```python
from build123d import *

# Parameters (mm, degrees)
EXTRUDE_1_DEPTH     = 11
SKETCH_2_R          = 1.5
SKETCH_2_R_2        = 4
CUT_EXTRUDE_1_DEPTH = 10
SKETCH_4_R          = 4
SKETCH_4_R_2        = 1.1
CUT_EXTRUDE_4_DEPTH = 20
SKETCH_5_W          = 18.664238265
SKETCH_5_H          = 20
CUT_EXTRUDE_5_DEPTH = 20
SKETCH_6_W          = 87
SKETCH_6_H          = 5
EXTRUDE_2_DEPTH     = 11
CUT_EXTRUDE_6_DEPTH = 11


with BuildPart() as part:
    # 草图1 → 凸台-拉伸1 (new body)
    with BuildSketch(Plane(origin=(0, 0, 0), x_dir=(1, 0, 0), z_dir=(0, 1, 0))):
        with BuildLine():
            Line((-41.199983302, 20), (78.800016698, 20))
            Line((78.800016698, 20), (78.800016698, 0))
            Line((78.800016698, 0), (-41.199983302, 0))
            ThreePointArc((-41.199983302, 0), (-51.199983302, 10), (-41.199983302, 20))
        make_face()
    extrude(amount=EXTRUDE_1_DEPTH)

    # 草图2 → 切除-拉伸1 (cut)
    with BuildSketch(Plane(origin=(0, 11, 0), x_dir=(1, 0, 0), z_dir=(0, 1, 0))):
        with Locations(Location((-48.199983302, 10, 0), (0, 0, 270))):
            Circle(SKETCH_2_R)
        with BuildLine():
            ThreePointArc((-39.699983302, 17), (-40.13932313, 18.060660172), (-41.199983302, 18.5))
            Line((-41.199983302, 18.5), (-41.199983302, 17))
            Line((-41.199983302, 17), (-41.199983302, 15.5))
            ThreePointArc((-41.199983302, 15.5), (-40.13932313, 15.939339828), (-39.699983302, 17))
        make_face()
        with BuildLine():
            Line((-41.199983302, 17), (-41.199983302, 18.5))
            ThreePointArc((-41.199983302, 18.5), (-42.699983302, 17), (-41.199983302, 15.5))
            Line((-41.199983302, 15.5), (-41.199983302, 17))
        make_face()
        with BuildLine():
            ThreePointArc((-39.699983302, 3), (-40.13932313, 4.060660172), (-41.199983302, 4.5))
            Line((-41.199983302, 4.5), (-41.199983302, 3))
            Line((-41.199983302, 3), (-41.199983302, 1.5))
            ThreePointArc((-41.199983302, 1.5), (-40.13932313, 1.939339828), (-39.699983302, 3))
        make_face()
        with BuildLine():
            Line((-41.199983302, 3), (-41.199983302, 4.5))
            ThreePointArc((-41.199983302, 4.5), (-42.699983302, 3), (-41.199983302, 1.5))
            Line((-41.199983302, 1.5), (-41.199983302, 3))
        make_face()
        with Locations(Location((-41.199983302, 10, 0), (0, 0, 270))):
            Circle(SKETCH_2_R_2)
    extrude(amount=-CUT_EXTRUDE_1_DEPTH, mode=Mode.SUBTRACT)

    # 草图4 → 切除-拉伸4 (cut)
    with BuildSketch(Plane(origin=(0, 11, 0), x_dir=(1, 0, 0), z_dir=(0, 1, 0))):
        with Locations(Location((69.300016698, 10, 0), (0, 0, 270))):
            Circle(SKETCH_4_R)
        with Locations(Location((76.7246379, 17.424621202, 0), (0, 0, 270))):
            Circle(SKETCH_4_R_2)
        with Locations(Location((62.300016698, 10, 0), (0, 0, 270))):
            Circle(SKETCH_4_R_2)
        with Locations(Location((76.7246379, 2.575378798, 0), (0, 0, 270))):
            Circle(SKETCH_4_R_2)
        with Locations(Location((61.875395496, 2.575378798, 0), (0, 0, 270))):
            Circle(SKETCH_4_R_2)
        with Locations(Location((61.875395496, 17.424621202, 0), (0, 0, 270))):
            Circle(SKETCH_4_R_2)
        with Locations(Location((69.300016698, 17, 0), (0, 0, 270))):
            Circle(SKETCH_4_R_2)
        with Locations(Location((76.300016698, 10, 0), (0, 0, 270))):
            Circle(SKETCH_4_R_2)
        with Locations(Location((69.300016698, 3, 0), (0, 0, 270))):
            Circle(SKETCH_4_R_2)
    extrude(amount=-CUT_EXTRUDE_4_DEPTH, mode=Mode.SUBTRACT)

    # 草图5 → 切除-拉伸5 (cut)
    with BuildSketch(Plane.XZ):
        with Locations((-44.032102435, -10)):
            Rectangle(SKETCH_5_W, SKETCH_5_H)
    extrude(amount=-CUT_EXTRUDE_5_DEPTH, mode=Mode.SUBTRACT)

    # 草图6 → 凸台-拉伸2 (add)
    with BuildSketch(Plane(origin=(0, 11, 0), x_dir=(1, 0, 0), z_dir=(0, 1, 0))):
        Polygon((78.800016698, 20), (52.300016698, 25), (52.300016698, 20), align=None)
        Polygon((78.800016698, 0), (52.300016698, 0), (52.300016698, -5), align=None)
        with Locations((8.800016698, 22.5)):
            Rectangle(SKETCH_6_W, SKETCH_6_H)
        with Locations((8.800016698, -2.5)):
            Rectangle(SKETCH_6_W, SKETCH_6_H)
    extrude(amount=-EXTRUDE_2_DEPTH)

    # 草图7 → 切除-拉伸6 (cut)
    with BuildSketch(Plane(origin=(0, 11, 0), x_dir=(1, 0, 0), z_dir=(0, 1, 0))):
        with BuildLine():
            Line((23.300016698, 17.5), (25.300016698, 17.5))
            Line((25.300016698, 17.5), (25.300016698, 15.5))
            ThreePointArc((25.300016698, 15.5), (26.71423026, 16.085786438), (27.300016698, 17.5))
            ThreePointArc((27.300016698, 17.5), (25.300016698, 19.5), (23.300016698, 17.5))
        make_face()
        with BuildLine():
            Line((25.300016698, 15.5), (25.300016698, 17.5))
            Line((25.300016698, 17.5), (23.300016698, 17.5))
            ThreePointArc((23.300016698, 17.5), (23.885803136, 16.085786438), (25.300016698, 15.5))
        make_face()
        with BuildLine():
            ThreePointArc((27.300016698, 2.5), (26.71423026, 3.914213562), (25.300016698, 4.5))
            Line((25.300016698, 4.5), (25.300016698, 2.5))
            Line((25.300016698, 2.5), (23.300016698, 2.5))
            ThreePointArc((23.300016698, 2.5), (25.300016698, 0.5), (27.300016698, 2.5))
        make_face()
        with BuildLine():
            Line((25.300016698, 2.5), (25.300016698, 4.5))
            ThreePointArc((25.300016698, 4.5), (23.885803136, 3.914213562), (23.300016698, 2.5))
            Line((23.300016698, 2.5), (25.300016698, 2.5))
        make_face()
        with BuildLine():
            ThreePointArc((-14.699983302, 15.5), (-13.28576974, 16.085786438), (-12.699983302, 17.5))
            Line((-12.699983302, 17.5), (-14.699983302, 17.5))
            Line((-14.699983302, 17.5), (-14.699983302, 15.5))
        make_face()
        with BuildLine():
            Line((-14.699983302, 17.5), (-12.699983302, 17.5))
            ThreePointArc((-12.699983302, 17.5), (-16.114196864, 18.914213562), (-14.699983302, 15.5))
            Line((-14.699983302, 15.5), (-14.699983302, 17.5))
        make_face()
        with BuildLine():
            ThreePointArc((-14.699983302, 4.5), (-16.114196864, 1.085786438), (-12.699983302, 2.5))
            Line((-12.699983302, 2.5), (-14.699983302, 2.5))
            Line((-14.699983302, 2.5), (-14.699983302, 4.5))
        make_face()
        with BuildLine():
            Line((-14.699983302, 2.5), (-12.699983302, 2.5))
            ThreePointArc((-12.699983302, 2.5), (-13.28576974, 3.914213562), (-14.699983302, 4.5))
            Line((-14.699983302, 4.5), (-14.699983302, 2.5))
        make_face()
    extrude(amount=-CUT_EXTRUDE_6_DEPTH, mode=Mode.SUBTRACT)


solid = part.part
```
Model file for the job. Use its own axes, mm. Give positions to 0.01 mm unless a question says otherwise; leave off trailing zeros. Loops run counter-clockwise (first coordinate to the right, second up) from the corner with the lowest first, then second, coordinate; pieces in that order, holes last. Notation, with made-up numbers: (-9, 25) -> (45, 25) arc R25 ccw to (45, 48) -> close; hole circle Ø2 at (22.25, 36). An arc over 180 degrees is marked (long way). Use CSV: the item, a comma, the result in double quotes. Start each with the question number.
1) Wall check: line 1 (X direction, y = 6, z = -10); line 2 (X direction, y = 3, z = -17); line 3 (Z direction, x = -16, y = 6.25). Give the ranges that are in metal, low to high.
2) Flat gauge pin, fed straight in: pin 1 Ø3.5 at (x, z) = (-14.7, -17.5) entering from +Y. Where does the tip first touch, or does it go through?
3) Slice it at C-C on z = 3.25. Give the cut face in (x, y).
4) Mould opens along X. For faces 1 (the flat face through (8, 6, -25)), 2 (the flat face through (-34.7, 6, -10)), 3 (the flat face through (65.365, 5.577, 2.535)), 4 (the cylindrical face through (68.324, 5.577, -2.492)) say: released by +X, released by -X, zero draft, split by the parting line, or undercut.
5) Slice it at D-D on z = -23. Give the cut face in (x, y).
6) Slice it at A-A on z = -10. Give the cut face in (x, y), plus the area to 3 significant figures.
7) Slice it at B-B on y = 5.25. Give the number of separate pieces and of enclosed holes in the cut face, plus the area to 3 significant figures.
Computed values:
1,line 1,"x = -34.7 to 61.2, 63.4 to 65.3, 73.3 to 75.2, 77.4 to 78.8"
1,line 2,"x = -34.7 to -16.64, -12.76 to 23.36, 27.24 to 60.86, 62.89 to 68.2, 70.4 to 75.71, 77.74 to 78.8"
1,line 3,"z = -25 to -19.02, -15.98 to -4.02, -0.98 to 5"
2,pin 1,"passes through"
3,outline,"(-34.7, 0) -> (61.58, 0) -> (61.58, 11) -> (-34.7, 11) -> close"
4,face 1,"zero draft"
4,face 2,"released by -X"
4,face 3,"released by +X"
4,face 4,"undercut"
5,outline,"(-34.7, 0) -> (62.9, 0) -> (62.9, 11) -> (-34.7, 11) -> close"
6,outline,"(-34.7, 0) -> (61.2, 0) -> (61.2, 11) -> (-34.7, 11) -> close; (63.4, 0) -> (65.3, 0) -> (65.3, 11) -> (63.4, 11) -> close; (73.3, 0) -> (75.2, 0) -> (75.2, 11) -> (73.3, 11) -> close; (77.4, 0) -> (78.8, 0) -> (78.8, 11) -> (77.4, 11) -> close"
6,area,"1,110 mm^2"
7,separate pieces,"1"
7,enclosed holes,"13"
7,area,"3,140 mm^2"
